Read the model definition and answer for the solid it produces. Units are mm, in the model's axes. A direction names the side the tool comes from. Give positions to 0.01 mm unless a question says otherwise; leave off trailing zeros. Loops run counter-clockwise (first coordinate to the right, second up) from the corner with the lowest first, then second, coordinate; pieces in that order, holes last. Notation, with made-up numbers: (51, 16.5) -> (93, 16.5) arc R5 ccw to (93, 24.5) -> close; hole circle Ø4 at (23.25, 36.5). An arc over 180 degrees is marked (long way). Return JSON: item names as keys, results as strings. Group by question number.
from build123d import *

# Parameters (mm, degrees)
SKETCH1_R           = 1.75
BOSS_EXTRUDE1_DEPTH = 4
SKETCH2_W           = 3
SKETCH2_H           = 3
CUT_EXTRUDE1_DEPTH  = 21.396078054
SKETCH3_R           = 2
CUT_EXTRUDE2_DEPTH  = 1


with BuildPart() as part:
    # Sketch1 → Boss-Extrude1 (new body)
    with BuildSketch(Plane.XY):
        with BuildLine():
            Line((-8, 6), (-8, -6))
            Line((-8, -6), (-12, -6))
            ThreePointArc((-12, -6), (0, -16), (12, -6))
            Line((12, -6), (8, -6))
            Line((8, -6), (8, 6))
            ThreePointArc((8, 6), (0, 14), (-8, 6))
        make_face()
        with Locations((0, 5)):
            Circle(SKETCH1_R, mode=Mode.SUBTRACT)
        with Locations((0, -5)):
            Circle(SKETCH1_R, mode=Mode.SUBTRACT)
    extrude(amount=BOSS_EXTRUDE1_DEPTH)

    # Sketch2 → Cut-Extrude1 (cut, through all)
    with BuildSketch(Plane.XY.offset(4)):
        with Locations((0, 9.5)):
            Rectangle(SKETCH2_W, SKETCH2_H)
        with Locations((0, -9.5)):
            Rectangle(SKETCH2_W, SKETCH2_H)
    extrude(amount=-CUT_EXTRUDE1_DEPTH, mode=Mode.SUBTRACT)

    # Sketch3 → Cut-Extrude2 (cut)
    with BuildSketch(Plane.XY.offset(4)):
        with Locations((0, 5)):
            Circle(SKETCH3_R)
    extrude(amount=-CUT_EXTRUDE2_DEPTH, mode=Mode.SUBTRACT)


solid = part.part
1. Section A-A on y = -5 is taken. Determine the outline of the cut face in (x, z).
2. Which of the six approach directions +Z, -Z, +X, -X, +Y, -Y give full straight-line access (tool end or side, diameter ignored) to faces 1 (the flat face through (10, -6, 2)), 2 (the flat face through (-10, -6, 2)), 3 (the flat face through (0, -8, 2))?
3. Straight lines are drawn through the part: line 1 (Y direction, x = 0, z = 3.7); line 2 (Y direction, x = 0, z = 2.65); line 3 (X direction, y = -0.5, z = 2.55). For each, find the intervals that lie inside material, in ascending order. Write a range as from..to.
4. Flat-ended cylindrical pins translate along their axes: pin 1 Ø1 at (y, z) = (-3.5, 1) entering from -X; pin 2 Ø1.5 at (y, z) = (9, 2) entering from -X; pin 3 Ø1.2 at (y, z) = (0.5, 2.5) entering from +X. Find the tip coordinate at first contact, or state that the pin passes through.
5. Section D-D on z = 3.45 is taken. Determine the outline of the cut face in (x, y), then the cut area to 3 significant figures.
6. Section B-B on x = 0 is taken. Determine the outline of the cut face in (y, z), then the cut area to 3 significant figures.
7. Determine the mould class of faces 4 (the cylindrical face through (-0.38, 3.29, 1.48)), 5 (the flat face through (0, 11, 2)), 6 (the flat face through (8, 0, 2)), 7 (the cylindrical face through (0, -16, 2)) for opening direction X: pulls with the +X half, pulls with the -X half, needs draft (parallel to the pull), parting line crosses it, or undercut.
8. Section C-C on z = 0.9 is taken. Determine the outline of the cut face in (x, y).
Completed:
{
 "1": {"outline": "(-8, 0) -> (-1.75, 0) -> (-1.75, 4) -> (-8, 4) -> close; (1.75, 0) -> (8, 0) -> (8, 4) -> (1.75, 4) -> close"},
 "2": {"face 1": "+Z, -Z, +X, +Y", "face 2": "+Z, -Z, -X, +Y", "face 3": "+Z, -Z"},
 "3": {"line 1": "y = -16..-11, -8..-6.75, -3.25..3, 7..8, 11..14", "line 2": "y = -16..-11, -8..-6.75, -3.25..3.25, 6.75..8, 11..14", "line 3": "x = -8..8"},
 "4": {"pin 1": "stops at x = -8", "pin 2": "stops at x = -7.68", "pin 3": "stops at x = 8"},
 "5": {"outline": "(-12, -6) arc R12.2 ccw to (12, -6) -> (8, -6) -> (8, 6) arc R8 ccw to (-8, 6) -> (-8, -6) -> close; hole circle Ø4 at (0, 5); hole circle Ø3.5 at (0, -5); hole (-1.5, -11) -> (1.5, -11) -> (1.5, -8) -> (-1.5, -8) -> close; hole (-1.5, 8) -> (1.5, 8) -> (1.5, 11) -> (-1.5, 11) -> close", "area": "433 mm²"},
 "6": {"outline": "(-16, 0) -> (-11, 0) -> (-11, 4) -> (-16, 4) -> close; (-8, 0) -> (-6.75, 0) -> (-6.75, 4) -> (-8, 4) -> close; (-3.25, 0) -> (3.25, 0) -> (3.25, 3) -> (3, 3) -> (3, 4) -> (-3.25, 4) -> close; (6.75, 0) -> (8, 0) -> (8, 4) -> (7, 4) -> (7, 3) -> (6.75, 3) -> close; (11, 0) -> (14, 0) -> (14, 4) -> (11, 4) -> close", "area": "67.5 mm²"},
 "7": {"face 4": "undercut", "face 5": "undercut", "face 6": "pulls with the +X half", "face 7": "parting line crosses it"},
 "8": {"outline": "(-12, -6) arc R12.2 ccw to (12, -6) -> (8, -6) -> (8, 6) arc R8 ccw to (-8, 6) -> (-8, -6) -> close; hole circle Ø3.5 at (0, -5); hole circle Ø3.5 at (0, 5); hole (-1.5, -11) -> (1.5, -11) -> (1.5, -8) -> (-1.5, -8) -> close; hole (-1.5, 8) -> (1.5, 8) -> (1.5, 11) -> (-1.5, 11) -> close"}
}
